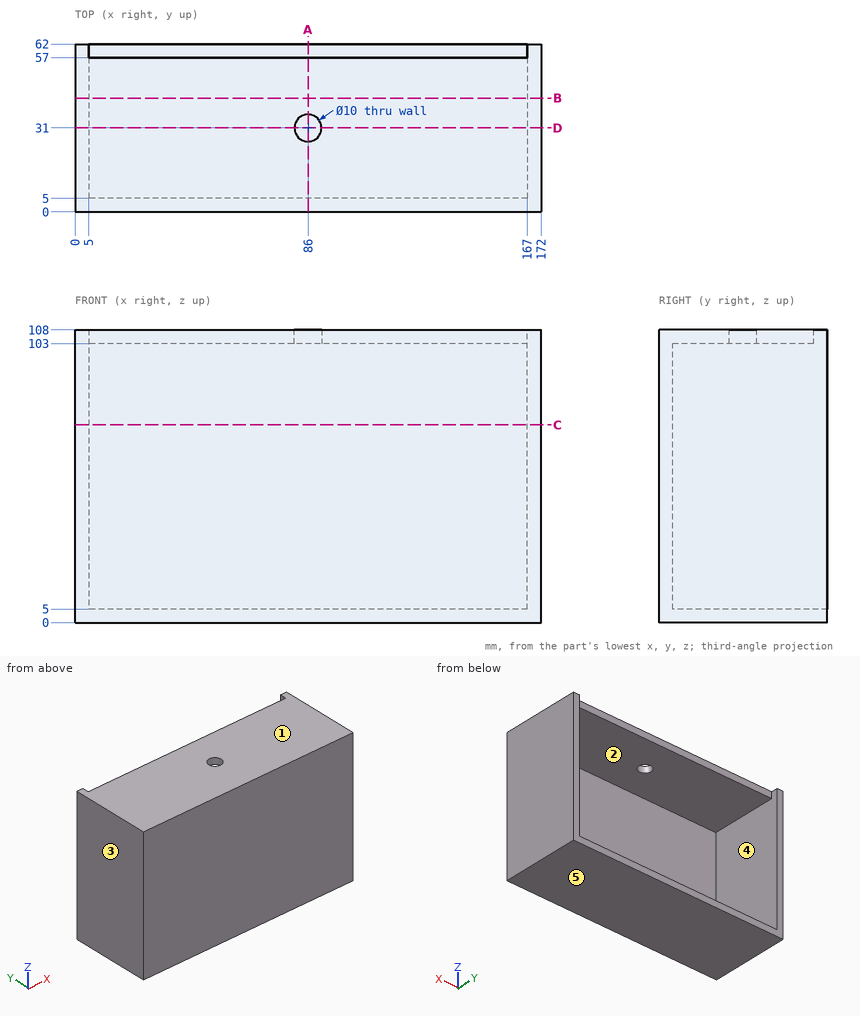
Can you work these out from the drawing? Everything is in mm from the part's minimum corner. A direction names the side the tool comes from. Give positions to 0.01 mm unless a question says otherwise; leave off trailing zeros. Write each loop counter-clockwise with the first axis right and the second up, starting at its lowest first coordinate (ties: lowest second). Pieces come first, ordered by that corner, then holes. Notation, with made-up numbers: M -4,7.5 L 53,7.5 A27 ccw 53,35.5 Z; hole C 24,84 d11. An arc over 180 degrees is marked long. Answer in a Markdown table with one row per item. Add a question column.
Item 1: Please list where these lines run through material, in increasing order: L1, parallel to X at y = 23.5, z = 54; L2, parallel to Z at x = 54, y = 6; L3, parallel to Y at x = 86, z = 106.
Item 2: Imagine slicing it at C-C, the plane z = 73. Write out the boundary of the cut face in (x, y).
Item 3: On a 3-axis mill with a long thin cutter (end or side, diameter ignored), from which of +Z, -Z, +X, -X, +Y, -Y can I reach the whole of each face in a straight line? I mean the marked faces 1 and 2. Say none if no direction works.
Item 4: Imagine slicing it at D-D, the plane y = 31. Write out the boundary of the cut face in (x, z).
Item 5: Imagine slicing it at A-A, the plane x = 86. Write out the boundary of the cut face in (y, z), plus the area to 4 significant figures.
Item 6: We'd pull the mould along Z, two halves only. Please class the marked faces 3, 4 and 5: released by +Z, released by -Z, zero draft, split by the parting line, or undercut.
Item 7: For pin 1 Ø6 at (x, z) = (60.5, 23) entering from +Y; pin 2 Ø5.5 at (x, z) = (88, 105) entering from +Y, each with a flat end and sliding along its axis, tell me the tip position at first contact or that it passes through.
Item 8: Imagine slicing it at B-B, the plane y = 42. Write out the boundary of the cut face in (x, z), plus the area to 3 significant figures.
Evaluation:
| question | item | result |
|---|---|---|
| 1 | L1 | x = 0 to 5, 167 to 172 |
| 1 | L2 | z = 0 to 5, 103 to 108 |
| 1 | L3 | y = 0 to 26, 36 to 57 |
| 2 | outline | M 0,0 L 172,0 L 172,62 L 167,62 L 167,5 L 5,5 L 5,62 L 0,62 Z |
| 3 | face 1 | +Z, +X, -X, +Y, -Y |
| 3 | face 2 | +Y |
| 4 | outline | M 0,0 L 172,0 L 172,108 L 91,108 L 91,103 L 167,103 L 167,5 L 5,5 L 5,103 L 81,103 L 81,108 L 0,108 Z |
| 5 | outline | M 0,0 L 62,0 L 62,5 L 5,5 L 5,103 L 26,103 L 26,108 L 0,108 Z; M 36,103 L 57,103 L 57,108 L 36,108 Z |
| 5 | area | 1,035 mm² |
| 6 | face 3 | zero draft |
| 6 | face 4 | undercut |
| 6 | face 5 | released by -Z |
| 7 | pin 1 | stops at y = 5 |
| 7 | pin 2 | stops at y = 57 |
| 8 | outline | M 0,0 L 172,0 L 172,108 L 0,108 Z; hole M 5,5 L 167,5 L 167,103 L 5,103 Z |
| 8 | area | 2,700 mm² |
